Check sheet for the modelled part. Datum: model origin and axes. Units: mm. Give positions to 0.01 mm unless a question says otherwise; leave off trailing zeros. Write each loop counter-clockwise with the first axis right and the second up, starting at its lowest first coordinate (ties: lowest second). Pieces come first, ordered by that corner, then holes. Notation, with made-up numbers: (-24.75, 51.5) - (-7.75, 51.5) arc R27 cw to (-7.75, 79.5) - close; hole circle Ø8 at (-31, 48.5). An arc over 180 degrees is marked (long way). Return JSON: item names as keys, results as strings. Group by question number.
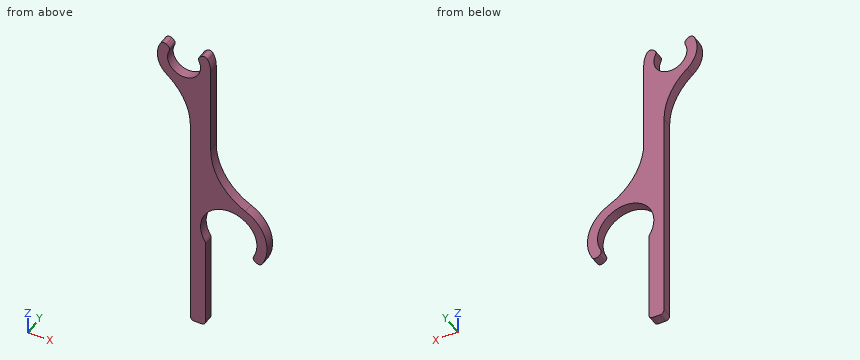
```python
from build123d import *

# Parameters (mm, degrees)
F1_DEPTH = 5
F2_R     = 2
F3_R     = 30.3991713246


with BuildPart() as f1:
    # F0 (on Front) → F1 (new body)
    with BuildSketch(Plane.XZ):
        with BuildLine():
            ThreePointArc((8.4325112108, -10.0903545369), (5.9438997073, -11.7299853482), (3.15, -12.7671453348))
            Line((3.15, -12.7671453348), (3.15, -88.05))
            ThreePointArc((3.15, -88.05), (3.6076950345, -83.915826859), (4.9586124402, -79.9818855189))
            ThreePointArc((4.9586124402, -79.9818855189), (8.3605698088, -75.0189025389), (13.15, -71.3766679995))
            Line((13.15, -71.3766679995), (13.15, 0))
            ThreePointArc((13.15, 0), (11.91238898, -5.569334681), (8.4325112108, -10.0903545369))
        make_face()
        with BuildLine():
            ThreePointArc((4.9586124402, -79.9818855189), (3.6076950345, -83.915826859), (3.15, -88.05))
            ThreePointArc((3.15, -88.05), (4.0247496309, -93.7333396106), (6.5680263629, -98.890594647))
            Line((6.5680263629, -98.890594647), (10.6637865844, -96.0227124653))
            ThreePointArc((10.6637865844, -96.0227124653), (22.05, -74.15), (33.4362134156, -96.0227124653))
            Line((33.4362134156, -96.0227124653), (37.5319736371, -98.890594647))
            ThreePointArc((37.5319736371, -98.890594647), (36.1951275757, -75.5150342694), (13.15, -71.3766679995))
            ThreePointArc((13.15, -71.3766679995), (8.3605698088, -75.0189025389), (4.9586124402, -79.9818855189))
        make_face()
        with BuildLine():
            ThreePointArc((6.5680263629, -98.890594647), (4.0247496309, -93.7333396106), (3.15, -88.05))
            Line((3.15, -88.05), (3.15, -141.95))
            Line((3.15, -141.95), (10.6637865844, -141.95))
            Line((10.6637865844, -141.95), (10.6637865844, -103.1352293338))
            ThreePointArc((10.6637865844, -103.1352293338), (8.4492978203, -101.1736770845), (6.5680263629, -98.890594647))
        make_face()
        with BuildLine():
            Line((10.6637865844, -96.0227124653), (6.5680263629, -98.890594647))
            ThreePointArc((6.5680263629, -98.890594647), (8.4492978203, -101.1736770845), (10.6637865844, -103.1352293338))
            Line((10.6637865844, -103.1352293338), (10.6637865844, -96.0227124653))
        make_face()
        with BuildLine():
            ThreePointArc((-10.4325964248, 8.0052127915), (-12.666067706, -3.5345761935), (-4.7800799709, -12.2504422562))
            ThreePointArc((-4.7800799709, -12.2504422562), (-0.8550062548, -13.1221745265), (3.15, -12.7671453348))
            ThreePointArc((3.15, -12.7671453348), (5.9438997073, -11.7299853482), (8.4325112108, -10.0903545369))
            ThreePointArc((8.4325112108, -10.0903545369), (11.91238898, -5.569334681), (13.15, 0))
            ThreePointArc((13.15, 0), (12.4521312029, 4.2269289687), (10.4325964248, 8.0052127915))
            Line((10.4325964248, 8.0052127915), (6.4658297234, 4.9614056464))
            ThreePointArc((6.4658297234, 4.9614056464), (0, -8.15), (-6.4658297234, 4.9614056464))
            Line((-6.4658297234, 4.9614056464), (-10.4325964248, 8.0052127915))
        make_face()
    extrude(amount=F1_DEPTH)

    # F2
    f2_edges = [f1.edges().sort_by_distance(p)[0] for p in [
        (6.46583, -2.5, 4.961406),
        (-6.46583, -2.5, 4.961406),
        (-10.432596, -2.5, 8.005213),
        (10.663787, -2.5, -96.022712),
        (33.436213, -2.5, -96.022712),
        (37.531974, -2.5, -98.890595),
        (3.15, -2.5, -141.95),
        (10.663787, -2.5, -141.95),
        (10.432596, -2.5, 8.005213),
    ]]
    fillet(f2_edges, radius=F2_R)

    # F3
    f3_edges = [f1.edges().sort_by_distance(p)[0] for p in [
        (3.15, -2.5, -12.767145),
        (13.15, -2.5, -71.376668),
    ]]
    fillet(f3_edges, radius=F3_R)


solid = f1.part
```
Item 1: Section check C-C on z = -67. Record the cut outline in (x, y).
Item 2: Material ranges on line 1 along X through (y, z) = (-3.55, -88.05); line 2 along X through (y, z) = (-3.75, -101); line 3 along X through (y, z) = (-2.2, 0), recorded low to high. Write a range as from..to.
Item 3: Section check A-A on z = -88.05. Record the cut outline in (x, y).
Item 4: Section check B-B on x = 22. Record the cut outline in (y, z).
Item 5: Depth check by flat-ended pin: pin 1 (8 mm diameter, centred on x = 14.5, z = -46, fed in from +Y); pin 2 (3 mm diameter, centred on x = -6, y = -1.5, fed in from -Z); pin 3 (2 mm diameter, centred on y = -3, z = -32, fed in from +X); pin 4 (2.5 mm diameter, centred on y = -1.5, z = -120.5, fed in from +X). Enter the tip coordinate at first touch or a pass-through.
Reply:
{
 "1": {"outline": "(3.15, -5) - (24.04, -5) - (24.04, 0) - (3.15, 0) - close"},
 "2": {"line 1": "3.15..8.15, 35.95..40.95", "line 2": "3.15..10.66", "line 3": "-13.15..-8.15, 8.15..13.15"},
 "3": {"outline": "(3.15, -5) - (8.15, -5) - (8.15, 0) - (3.15, 0) - close; (35.95, -5) - (40.95, -5) - (40.95, 0) - (35.95, 0) - close"},
 "4": {"outline": "(-5, -74.15) - (0, -74.15) - (0, -65.13) - (-5, -65.13) - close"},
 "5": {"pin 1": "y = 0", "pin 2": "z = -13.81", "pin 3": "x = 13.15", "pin 4": "x = 10.66"}
}
